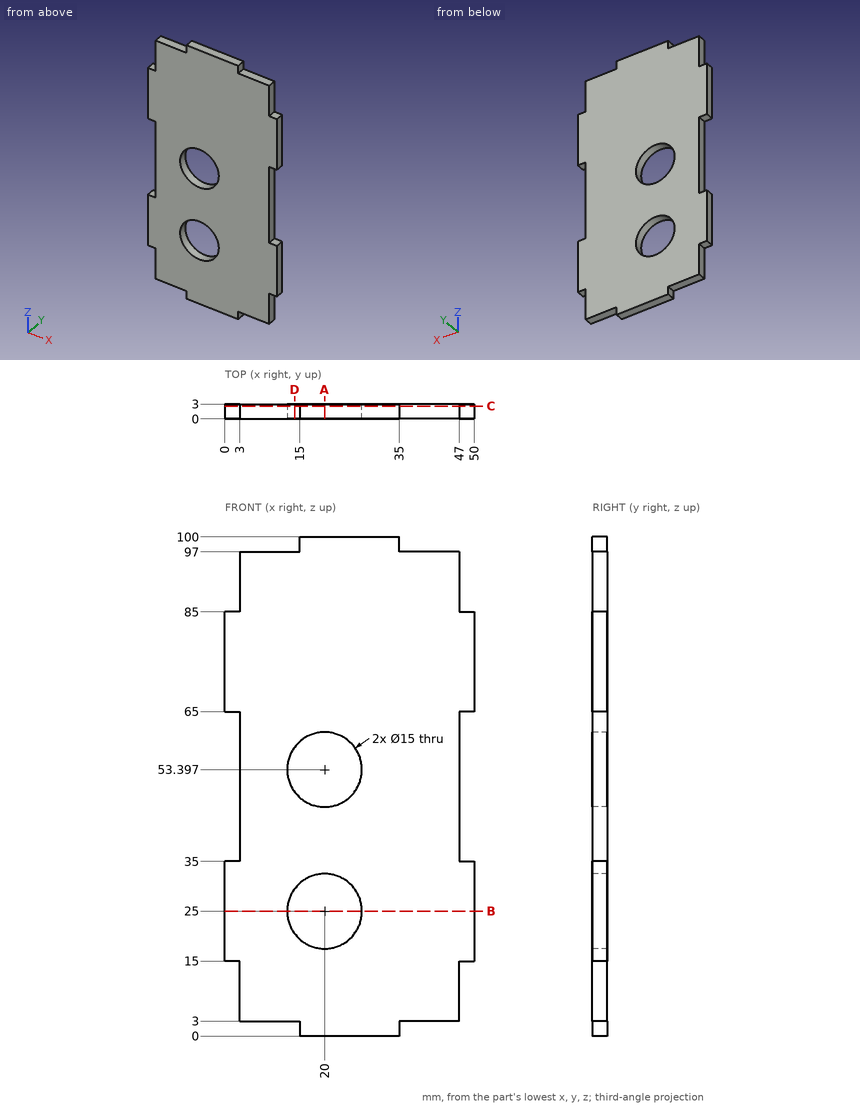
Job drawing, mm, ordinate dimensions from the low corner. One solid piece. Round coordinates to 2 decimals unless told otherwise and drop trailing zeros. Loops run counter-clockwise (first coordinate to the right, second up) from the corner with the lowest first, then second, coordinate; pieces in that order, holes last.
Item 1: Drill centre lines: line 1 (Z direction, x = 20, y = 2.3); line 2 (X direction, y = 1.05, z = 53.5); line 3 (Z direction, x = 25.5, y = 0.5). Where is each one in solid material? Low to high.
Item 2: Cut at A-A, the plane x = 20. Give the cut face in (y, z), then the cut area to 3 significant figures.
Item 3: Cut at B-B, the plane z = 25. Give the cut face in (x, y), then the cut area to 3 significant figures.
Item 4: Cut at D-D, the plane x = 14. Give the cut face in (y, z).
Item 5: Cut at C-C, the plane y = 2.55. State how many separate pieces and enclosed holes the cut face has, then the cut area to 3 significant figures.
Item 6: Drop flat-ended pins along their axis: P1, Ø0.9, axis at y = 1.5, z = 47.5, coming from the +X side; P2, Ø19.5, axis at x = 20, z = 25, coming from the -Y side; P3, Ø1.5, axis at x = 8.5, y = 2, coming from the +Z side; P4, Ø0.9, axis at x = 1.5, y = 1, coming from the -Z side. Give the stop position or say it passes through.
A:
1. line 1: z = 0 to 17.5, 32.5 to 45.9, 60.9 to 100
1. line 2: x = 3 to 12.5, 27.5 to 47
1. line 3: z = 0 to 19.9, 30.1 to 48.3, 58.5 to 100
2. outline: (0, 0) - (3, 0) - (3, 17.5) - (0, 17.5) - close; (0, 32.5) - (3, 32.5) - (3, 45.9) - (0, 45.9) - close; (0, 60.9) - (3, 60.9) - (3, 100) - (0, 100) - close
2. area: 210 mm2
3. outline: (0, 0) - (12.5, 0) - (12.5, 3) - (0, 3) - close; (27.5, 0) - (50, 0) - (50, 3) - (27.5, 3) - close
3. area: 105 mm2
4. outline: (0, 3) - (3, 3) - (3, 20.5) - (0, 20.5) - close; (0, 29.5) - (3, 29.5) - (3, 48.9) - (0, 48.9) - close; (0, 57.9) - (3, 57.9) - (3, 97) - (0, 97) - close
5. separate pieces: 1
5. enclosed holes: 2
5. area: 4,140 mm2
6. P1: stops at x = 47
6. P2: stops at y = 0
6. P3: stops at z = 97
6. P4: stops at z = 15
